The model under review builds one solid part; all positions refer to its coordinate system, in mm. Face numbers are marked on the shaded views. A direction names the side the tool comes from. Give positions to 0.01 mm unless a question says otherwise; leave off trailing zeros. Loops run counter-clockwise (first coordinate to the right, second up) from the corner with the lowest first, then second, coordinate; pieces in that order, holes last. Notation, with made-up numbers: M 18.25,-27 L 72.25,-27 A8 ccw 72.25,-20 Z; hole C -27.5,23 d1. An arc over 180 degrees is marked long. One line per item, written item: value. Start each with the question number.
Q1. We need section D-D on z = 3.05. Write out the cut boundary in (x, y), plus the area to 3 significant figures.
Q2. We need section A-A on z = 0.55. Write out the cut boundary in (x, y).
Q3. To check wall thickness, follow line 1 along X through (y, z) = (27, 4); line 2 along Y through (x, z) = (9, 0.6); line 3 along X through (y, z) = (-2, 1.2). State the ranges of each line that lie inside material, in increasing order. Write a range as from..to.
Q4. For the marked faces 5 and 6, list the 3-axis set-ups (+Z, -Z, +X, -X, +Y, -Y) from which the entire face can be reached by the end or side of a thin tool; tool diameter is ignored.
Q5. For pin 1 (1.3 mm diameter, centred on y = 32, z = 3.5, fed in from +X); pin 2 (1.5 mm diameter, centred on y = -7.5, z = 2.5, fed in from -X); pin 3 (1.2 mm diameter, centred on y = -9, z = 0.5, fed in from -X); pin 4 (6 mm diameter, centred on x = 13.5, y = 19, fed in from -Z), all flat-tipped, find the tip position at first contact; note any pin that passes through.
Q6. Mouldability with a two-part tool opening along Y and no side actions: class the marked faces 1, 2, 3 and 4 as released by +Y, released by -Y, zero draft, split by the parting line, or undercut.
Q7. We need section C-C on x = -2. Write out the cut boundary in (y, z), plus the area to 3 significant figures.
Q8. We need section B-B on y = 32. Write out the cut boundary in (x, z), plus the area to 3 significant figures.
```python
from build123d import *

# Parameters (mm, degrees)
F0_W     = 9.141622
F0_H     = 3.656581
F1_DEPTH = 4.5
F3_DEPTH = 2
F4_SIZE  = 3
F5_R     = 1


with BuildPart() as f1:
    # F0 (on Top) → F1 (new body)
    with BuildSketch(Plane.XY):
        Polygon((10, 36.911765), (-10, 36.911765), (-15, 26.911765), (-20, 6.911765), (-10, -13.088235), (-5.3, -13.088235), (-5.3, -7.788235), (6.632093, 6.465869), (12.109291, 1.639867), (5.3, -6.088235), (5.3, -13.088235), (10, -13.088235), (20, 6.911765), (15, 26.911765), align=None)
        with Locations((0, 31.958237)):
            Rectangle(F0_W, F0_H, mode=Mode.SUBTRACT)
    extrude(amount=F1_DEPTH)

    # F2 (on face) → F3 (join)
    with BuildSketch(Plane.XY.offset(4.5)):
        Polygon((-5.3, -7.788235), (-5.3, -13.088235), (5.3, -13.088235), (5.3, -6.088235), (12.109291, 1.639867), (6.632093, 6.465869), align=None)
    extrude(amount=-F3_DEPTH)

    # F4
    f4_edges = [f1.edges().sort_by_distance(p)[0] for p in [
        (15, -3.088235, 4.5),
        (17.5, 16.911765, 4.5),
        (-15, -3.088235, 4.5),
        (-17.5, 16.911765, 4.5),
        (-12.5, 31.911765, 4.5),
        (0, 36.911765, 4.5),
        (12.5, 31.911765, 4.5),
    ]]
    chamfer(f4_edges, length=F4_SIZE)

    # F5
    f5_edges = [f1.edges().sort_by_distance(p)[0] for p in [
        (4.570811, 30.129947, 2.25),
        (-4.570811, 30.129947, 2.25),
        (-4.570811, 33.786528, 2.25),
        (4.570811, 33.786528, 2.25),
    ]]
    fillet(f5_edges, radius=F5_R)


solid = f1.part
```
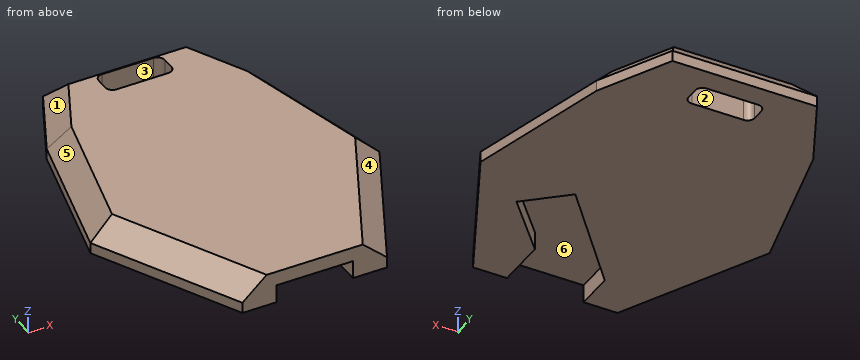
Solved:
1. outline: M -18.36,7.09 L -8.27,-13.09 L 8.27,-13.09 L 18.36,7.09 L 13.54,26.37 L 9.04,35.36 L -9.04,35.36 L -13.54,26.37 Z; hole M -4.57,31.13 A1 ccw -3.57,30.13 L 3.57,30.13 A1 ccw 4.57,31.13 L 4.57,32.79 A1 ccw 3.57,33.79 L -3.57,33.79 A1 ccw -4.57,32.79 Z
1. area: 1,320 mm2
2. outline: M -20,6.91 L -10,-13.09 L -5.3,-13.09 L -5.3,-7.79 L 6.63,6.47 L 12.11,1.64 L 5.3,-6.09 L 5.3,-13.09 L 10,-13.09 L 20,6.91 L 15,26.91 L 10,36.91 L -10,36.91 L -15,26.91 Z; hole M -4.57,31.13 A1 ccw -3.57,30.13 L 3.57,30.13 A1 ccw 4.57,31.13 L 4.57,32.79 A1 ccw 3.57,33.79 L -3.57,33.79 A1 ccw -4.57,32.79 Z
3. line 1: -12.16..12.16
3. line 2: -13.09..-1.89, 4.38..36.91
3. line 3: -15.54..-0.45, 8.9..15.54
4. face 5: +Z, -X, +Y
4. face 6: -Z
5. pin 1: x = 11.02
5. pin 2: x = -12.59
5. pin 3: x = -12.34
5. pin 4: z = 0
6. face 1: released by +Y
6. face 2: undercut
6. face 3: undercut
6. face 4: released by -Y
7. outline: M -13.09,2.5 L -3.85,2.5 L -3.85,0 L 30.13,0 L 30.13,4.5 L -13.09,4.5 Z; M 33.79,0 L 36.91,0 L 36.91,1.5 L 33.91,4.5 L 33.79,4.5 Z
7. area: 181 mm2
8. outline: M -12.46,0 L -4.57,0 L -4.57,4.5 L -9.1,4.5 L -12.46,1.5 Z; M 4.57,0 L 12.46,0 L 12.46,1.5 L 9.1,4.5 L 4.57,4.5 Z
8. area: 60.9 mm2
